Source: CAD feature listing. Evaluate the final solid. Frame: model axes, mm. A direction names the side the tool comes from. Coordinates: 2 decimals unless noted, no trailing zeros. Write each loop counter-clockwise with the first axis right and the second up, starting at its lowest first coordinate (ties: lowest second). Pieces come first, ordered by that corner, then holes. Notation, with made-up numbers: M 45.25,36 L 64.25,36 A12 cw 64.25,59 Z; hole C 12.25,-8.75 d6. An arc over 180 degrees is marked long. Write item = value, one per line. Start each with the question number.
1. Section query D-D (z = 30). Output: boundary loops of the cut face in (x, y).
2. Access query for faces 1 (the face through (0, -23, 13.5)), 2 (the face through (0, -23, 8)), 3 (the face through (-0.85, 23, 9)). Directions: +Z, -Z, +X, -X, +Y, -Y. A direction counts if a zero-diameter tool reaches every point of the face in a straight line with its end or side. Return the directions, or none.
3. Section query B-B (z = 9.5). Output: boundary loops of the cut face in (x, y), then the cut area to 3 significant figures.
4. Pin query (flat end, axial travel): pin 1 Ø8 at (x, y) = (-7, 0) entering from -Z; pin 2 Ø1.9 at (x, y) = (-0.5, 22.5) entering from -Z; pin 3 Ø6.5 at (x, y) = (-5.5, 25) entering from -Z. Return the tip coordinate at first contact, or that it passes through.
5. Section query A-A (x = 5.5). Output: boundary loops of the cut face in (y, z).
6. Line query: line 1 along X through (y, z) = (-25, 11.9); line 2 along Y through (x, z) = (-5.5, 11.3); line 3 along Z through (x, y) = (-0.75, -5). Output: solid intervals per line, ascending.
7. Section query C-C (y = -12). Output: boundary loops of the cut face in (x, z), then the cut area to 3 significant figures.
```python
from build123d import *

# Parameters (mm, degrees)
SKETCH1_W           = 20
SKETCH1_H           = 40
BOSS_EXTRUDE1_DEPTH = 41.6
SKETCH2_R           = 3
SKETCH2_R_2         = 1.5
BOSS_EXTRUDE2_DEPTH = 4
BOSS_EXTRUDE3_START = -13.5
BOSS_EXTRUDE3_DEPTH = 3
SKETCH5_W           = 1.7
SKETCH5_H           = 6
BOSS_EXTRUDE4_DEPTH = 2.5


with BuildPart() as part:
    # Sketch1 → Boss-Extrude1 (new body)
    with BuildSketch(Plane.XY):
        Rectangle(SKETCH1_W, SKETCH1_H)
    extrude(amount=BOSS_EXTRUDE1_DEPTH)

    # Sketch2 → Boss-Extrude2 (add)
    with BuildSketch(Plane(origin=(0, 0, 0), x_dir=(-1, 0, 0), z_dir=(0, 0, -1))):
        with Locations((0, 10)):
            Circle(SKETCH2_R)
        with Locations((0, 10)):
            Circle(SKETCH2_R_2, mode=Mode.SUBTRACT)
    extrude(amount=BOSS_EXTRUDE2_DEPTH)

    # Sketch3 → Boss-Extrude3 (add)
    with BuildSketch(Plane(origin=(0, 0, 0), x_dir=(-1, 0, 0), z_dir=(0, 0, -1)).offset(BOSS_EXTRUDE3_START)):
        with BuildLine():
            Line((-10, 27), (-10, 20))
            Line((-10, 20), (10, 20))
            Line((10, 20), (10, 27))
            Line((10, 27), (7, 27))
            ThreePointArc((7, 27), (7.736067977, 26.118033989), (8, 25))
            ThreePointArc((8, 25), (4.381966011, 22.763932023), (4, 27))
            Line((4, 27), (-4, 27))
            ThreePointArc((-4, 27), (-3.263932023, 26.118033989), (-3, 25))
            ThreePointArc((-3, 25), (-6.618033989, 22.763932023), (-7, 27))
            Line((-7, 27), (-10, 27))
        make_face()
        with BuildLine():
            Line((10, -20), (-10, -20))
            Line((-10, -20), (-10, -27))
            Line((-10, -27), (-7, -27))
            ThreePointArc((-7, -27), (-6.618033989, -22.763932023), (-3, -25))
            ThreePointArc((-3, -25), (-3.263932023, -26.118033989), (-4, -27))
            Line((-4, -27), (4, -27))
            ThreePointArc((4, -27), (4.381966011, -22.763932023), (8, -25))
            ThreePointArc((8, -25), (7.736067977, -26.118033989), (7, -27))
            Line((7, -27), (10, -27))
            Line((10, -27), (10, -20))
        make_face()
    extrude(amount=BOSS_EXTRUDE3_DEPTH)

    # Sketch5 → Boss-Extrude4 (add)
    with BuildSketch(Plane(origin=(0, 0, 10.5), x_dir=(-1, 0, 0), z_dir=(0, 0, -1))):
        with Locations((0, 23)):
            Rectangle(SKETCH5_W, SKETCH5_H)
        with Locations((0, -23)):
            Rectangle(SKETCH5_W, SKETCH5_H)
    extrude(amount=BOSS_EXTRUDE4_DEPTH)


solid = part.part
```
Results are:
q1.outline = M -10,-20 L 10,-20 L 10,20 L -10,20 Z
q2.face_1 = +Z, +X, -X, -Y
q2.face_2 = -Z, +X, -X, -Y
q2.face_3 = -Z, -X, +Y
q3.outline = M -10,-20 L -0.85,-20 L -0.85,-26 L 0.85,-26 L 0.85,-20 L 10,-20 L 10,20 L 0.85,20 L 0.85,26 L -0.85,26 L -0.85,20 L -10,20 Z
q3.area = 820 mm^2
q4.pin_1 = 0
q4.pin_2 = 8
q4.pin_3 = 10.5
q5.outline = M -22.5,10.5 L -20,10.5 L -20,0 L 20,0 L 20,10.5 L 22.5,10.5 L 22.5,13.5 L 20,13.5 L 20,41.6 L -20,41.6 L -20,13.5 L -22.5,13.5 Z
q6.line_1 = -10 to -8, -3 to 3, 8 to 10
q6.line_2 = -22.5 to 22.5
q6.line_3 = 0 to 41.6
q7.outline = M -10,0 L 10,0 L 10,41.6 L -10,41.6 Z
q7.area = 832 mm^2
